from build123d import *

# Parameters (mm, degrees)
CUT_EXTRUDE1_DEPTH = 4.2


with BuildPart() as part:
    # Sketch1 → Revolve1 (revolve)
    with BuildSketch(Plane.XY, mode=Mode.PRIVATE) as revolve1_sk:
        with BuildLine():
            Line((0, 25), (-5.7, 25))
            ThreePointArc((-5.7, 25), (-6.265685425, 24.765685425), (-6.5, 24.2))
            Line((-6.5, 24.2), (-6.5, 20))
            Line((-6.5, 20), (-4, 20))
            Line((-4, 20), (-4, 0))
            Line((-4, 0), (0, 0))
            Line((0, 0), (0, 25))
        make_face()
    revolve(revolve1_sk.sketch.rotate(Axis((0, 0, 0), (0, 1, 0)), 270), axis=Axis((0, 0, 0), (0, 1, 0)))

    # Sketch2 → Cut-Extrude1 (cut)
    with BuildSketch(Plane(origin=(0, 25, 0), x_dir=(1, 0, 0), z_dir=(0, 1, 0))):
        Polygon((0, 2.886751346), (-2.5, 1.443375673), (-2.5, -1.443375673), (0, -2.886751346), (2.5, -1.443375673), (2.5, 1.443375673), align=None)
    extrude(amount=-CUT_EXTRUDE1_DEPTH, mode=Mode.SUBTRACT)


solid = part.part
Model file for the job. Use its own axes, mm. A direction names the side the tool comes from. Give positions to 0.01 mm unless a question says otherwise; leave off trailing zeros. Order: outer loops, then holes, each group sorted by start corner. A loop starts at its lowest first (then second) coordinate and runs counter-clockwise, first axis right, second up. Notation, with made-up numbers: (3.5, 57.5) - (36.5, 57.5) arc R24 cw to (36.5, 78.5) - close; hole circle Ø8 at (32, 2). An arc over 180 degrees is marked (long way). Return JSON: item names as keys, results as strings.
1) Cut at B-B, the plane y = 23.75. Give the cut face in (x, z).
Geometry says:
{"outline": "circle Ø13 at (0, 0); hole (-2.5, -1.44) - (0, -2.89) - (2.5, -1.44) - (2.5, 1.44) - (0, 2.89) - (-2.5, 1.44) - close"}
2) Probe line 1 (X direction, y = 8, z = 0); line 2 (Y direction, x = 1.25, z = -4.75); line 3 (Y direction, x = 1.5, z = 0.25). List the from-to ranges inside material, lowest first. Write a range as from..to.
Geometry says:
{"line 1": "-4..4", "line 2": "20..25", "line 3": "0..20.8"}
3) Pull direction Z, two halves, no side cores. Call faces 1 (the cylindrical face through (3.905, 9.86, 0.867)), 2 (the flat face through (-3, 20, -3)), 3 (the flat face through (-1.267, 22.929, 2.155)): pulls with the +Z half, pulls with the -Z half, needs draft (parallel to the pull), parting line crosses it, or undercut.
Geometry says:
{"face 1": "parting line crosses it", "face 2": "needs draft", "face 3": "undercut"}
4) 3-axis set-ups, long thin cutter, end or side, ignore diameter. For faces 4 (the cylindrical face through (3.955, 22.071, 5.158)), 5 (the flat face through (1.267, 22.929, -2.155)): which of +Z, -Z, +X, -X, +Y, -Y reach the whole face in a straight line?
Geometry says:
{"face 4": "+Y, -Y", "face 5": "+Y"}
5) Flat gauge pins, fed straight in: P1, Ø5, axis at x = 0, y = 18.5, coming from the -Z side; P2, Ø3, axis at y = 8, z = -3.5, coming from the +X side; P3, Ø1.5, axis at x = 4, y = 9, coming from the +Z side; P4, Ø1, axis at y = 17.5, z = 3.5, coming from the -X side. Where does each tip first touch, or does it go through?
Geometry says:
{"P1": "z = -6.5", "P2": "x = 3.46", "P3": "z = 2.33", "P4": "x = -2.65"}
6) Cut at C-C, the plane y = 3.5. Give the cut face in (x, z).
Geometry says:
{"outline": "circle Ø8 at (0, 0)"}
7) Cut at A-A, the plane z = 0. Give the cut face in (x, y).
Geometry says:
{"outline": "(-6.5, 20) - (-4, 20) - (-4, 0) - (4, 0) - (4, 20) - (6.5, 20) - (6.5, 24.2) arc R0.8 ccw to (5.7, 25) - (2.5, 25) - (2.5, 20.8) - (-2.5, 20.8) - (-2.5, 25) - (-5.7, 25) arc R0.8 ccw to (-6.5, 24.2) - close"}
